Design review of the part built by this model. Coordinates are the model's own, in mm. A direction names the side the tool comes from. Give positions to 0.01 mm unless a question says otherwise; leave off trailing zeros. Loops run counter-clockwise (first coordinate to the right, second up) from the corner with the lowest first, then second, coordinate; pieces in that order, holes last. Notation, with made-up numbers: (63.5, 35) -> (111.5, 35) arc R33 ccw to (111.5, 67) -> close; hole circle Ø5 at (44.5, -12). An arc over 180 degrees is marked (long way). Answer as CSV lines item,"result".
from build123d import *

# Parameters (mm, degrees)
F0_W     = 12.7
F0_H     = 6.35
F1_DEPTH = 101.6
F2_R     = 1.5875
F2_R_2   = 3.175
F3_DEPTH = 6.351
F4_W     = 12.7
F4_H     = 1.5875
F5_DEPTH = 25.4


with BuildPart() as f1:
    # F0 (on Front) → F1 (new body)
    with BuildSketch(Plane.XZ):
        with Locations((6.35, 3.175)):
            Rectangle(F0_W, F0_H)
    extrude(amount=-F1_DEPTH)

    # F2 (on face) → F3 (cut, through all)
    with BuildSketch(Plane.XY.offset(6.35)):
        with Locations((6.35, 98.425)):
            Circle(F2_R)
        with Locations((6.35, 6.35)):
            Circle(F2_R_2)
    extrude(amount=-F3_DEPTH, mode=Mode.SUBTRACT)

    # F4 (on face) → F5 (cut)
    with BuildSketch(Plane(origin=(0, 101.6, 0), x_dir=(-1, 0, 0), z_dir=(0, 1, 0))):
        with Locations((-6.35, 5.55625)):
            Rectangle(F4_W, F4_H)
        with Locations((-6.35, 0.79375)):
            Rectangle(F4_W, F4_H)
    extrude(amount=-F5_DEPTH, mode=Mode.SUBTRACT)


solid = f1.part
Q1. For faces 1 (the flat face through (6, 101.6, 3)), 2 (the flat face through (6, 89, 1.588)), 3 (the flat face through (6, 76.2, 6)), list the 3-axis set-ups (+Z, -Z, +X, -X, +Y, -Y) from which the entire face can be reached by the end or side of a thin tool; tool diameter is ignored.
Filled sheet:
face 1,"+Z, -Z, +X, -X, +Y"
face 2,"-Z, +X, -X, +Y"
face 3,"+Z, +X, -X, +Y"
Q2. We need section A-A, the plane x = 6.35. State how many separate pieces and enclosed holes the cut face has, and give its area (3 significant figures).
Filled sheet:
separate pieces,"3"
enclosed holes,"0"
area,"514 mm^2"
Q3. We need section B-B, the plane y = 6.35. State the section outline as (x, z) points (3 decimals).
Filled sheet:
outline,"(0, 0) -> (3.175, 0) -> (3.175, 6.35) -> (0, 6.35) -> close; (9.525, 0) -> (12.7, 0) -> (12.7, 6.35) -> (9.525, 6.35) -> close"
Q4. Clearance check with a flat-ended pin moving along its axis: pin 1 Ø0.8 at (x, z) = (6.5, 6) entering from +Y. State where the tip first meets the part, or that it passes through.
Filled sheet:
pin 1,"stops at y = 76.2"
Q5. The part is to be moulded in two halves that separate along X. For faces 4 (the flat face through (12.7, 50, 3)), 5 (the flat face through (6, 0, 3)), 6 (the cylindrical face through (6.006, 96.875, 3.197)), 7 (the flat face through (0, 50, 3)), say which applies: pulls with the +X half, pulls with the -X half, needs draft (parallel to the pull), parting line crosses it, or undercut.
Filled sheet:
face 4,"pulls with the +X half"
face 5,"needs draft"
face 6,"undercut"
face 7,"pulls with the -X half"
Q6. We need section C-C, the plane x = 11. State the section outline as (y, z) points, and give its area (3 significant figures).
Filled sheet:
outline,"(0, 0) -> (76.2, 0) -> (76.2, 1.59) -> (101.6, 1.59) -> (101.6, 4.76) -> (76.2, 4.76) -> (76.2, 6.35) -> (0, 6.35) -> close"
area,"565 mm^2"
Q7. To check wall thickness, follow probe 1 along Y at (x, z) = (6.35, 3) (1 decimal); probe 2 along X at (y, z) = (6, 4); probe 3 along Y at (x, z) = (12, 1). State the ranges of each line that lie inside material, in increasing order. Write a range as from..to.
Filled sheet:
probe 1,"y = 0..3.2, 9.5..96.8, 100..101.6"
probe 2,"x = 0..3.19, 9.51..12.7"
probe 3,"y = 0..76.2"
